Work out the finished part from the listing and answer in its coordinate system (mm). A direction names the side the tool comes from. Give positions to 0.01 mm unless a question says otherwise; leave off trailing zeros. Loops run counter-clockwise (first coordinate to the right, second up) from the corner with the lowest first, then second, coordinate; pieces in that order, holes last. Notation, with made-up numbers: (-7, -1.5) - (33, -1.5) arc R22 cw to (33, 26.5) - close; hole circle Ø8 at (88.25, 13.5). An arc over 180 degrees is marked (long way). Use CSV: the item, a comma, the result in double quotes.
from build123d import *

# Parameters (mm, degrees)
SKETCH_1_W       = 20
SKETCH_1_H       = 10
BASEPLATE_DEPTH  = 1
HEM_OPEN_DEPTH   = 20
HEM_OPEN_2_DEPTH = 20


# Read off the part's stored shape, not the designer's step: Hem_open
# Sheet-metal steps are written as plain solids
with BuildPart() as part:
    # Sketch 1 → BasePlate (new body)
    with BuildSketch(Plane.XY):
        with Locations((10, 5)):
            Rectangle(SKETCH_1_W, SKETCH_1_H)
    extrude(amount=-BASEPLATE_DEPTH)

    # Hem_open outline → Hem_open (cut)
    with BuildSketch(Plane.YZ):
        with BuildLine():
            Line((10, 0), (9.914213562, 0))
            ThreePointArc((9.914213562, 0), (9.366025404, -0.724744871), (8.5, -1))
            Line((8.5, -1), (10, -1))
            Line((10, -1), (10, 0))
        make_face()
    extrude(amount=HEM_OPEN_DEPTH, mode=Mode.SUBTRACT)

    # Hem_open 2 outline → Hem_open 2 (add)
    with BuildSketch(Plane.YZ):
        with BuildLine():
            Line((5, 2), (5, 1))
            Line((5, 1), (8.5, 1))
            ThreePointArc((8.5, 1), (9, 0.5), (8.5, 0))
            Line((8.5, 0), (9.914213562, 0))
            ThreePointArc((9.914213562, 0), (9.724744871, 1.366025404), (8.5, 2))
            Line((8.5, 2), (5, 2))
        make_face()
    extrude(amount=HEM_OPEN_2_DEPTH)


solid = part.part
Item 1: Find the intervals of material crossed by line 1 (Z direction, x = 3.25, y = 5.5); line 2 (Z direction, x = 2.25, y = 8.75); line 3 (Z direction, x = 6.25, y = 1), in increasing order.
Determined:
line 1,"z = -1 to 0, 1 to 2"
line 2,"z = -0.98 to 0.07, 0.93 to 1.98"
line 3,"z = -1 to 0"
Item 2: For faces 1 (the flat face through (10, 7, 1)), 2 (the flat face through (9.9, 5, 1.5)), 3 (the flat face through (10, 7, 2)), determine the directions among +Z, -Z, +X, -X, +Y, -Y from which every point of the face is accessible in a straight line to the end or side of a thin tool.
Determined:
face 1,"+X, -X, -Y"
face 2,"+Z, +X, -X, -Y"
face 3,"+Z, +X, -X, +Y, -Y"
Item 3: A cutting plane is placed at B-B on x = 2.25. Determine the outline of the cut face in (y, z), and give its area (3 significant figures).
Determined:
outline,"(0, -1) - (8.5, -1) arc R1.5 ccw to (8.5, 2) - (5, 2) - (5, 1) - (8.5, 1) arc R0.5 cw to (8.5, 0) - (0, 0) - close"
area,"15.1 mm²"
Item 4: A cutting plane is placed at C-C on y = 1.5. Determine the outline of the cut face in (x, z).
Determined:
outline,"(0, -1) - (20, -1) - (20, 0) - (0, 0) - close"
Item 5: The mould has two halves that part along Z. Classify faces 4 (the flat face through (10, 4, -1)), 5 (the flat face through (10, 4, 0)), 6 (the flat face through (9.9, 0, -0.5)): pulls with the +Z half, pulls with the -Z half, needs draft (parallel to the pull), parting line crosses it, or undercut.
Determined:
face 4,"pulls with the -Z half"
face 5,"undercut"
face 6,"needs draft"
Item 6: A cutting plane is placed at A-A on y = 5.75. Determine the outline of the cut face in (x, z).
Determined:
outline,"(0, -1) - (20, -1) - (20, 0) - (0, 0) - close; (0, 1) - (20, 1) - (20, 2) - (0, 2) - close"
Item 7: A cutting plane is placed at D-D on z = 0.5. Determine the outline of the cut face in (x, y).
Determined:
outline,"(0, 9) - (20, 9) - (20, 10) - (0, 10) - close"
Item 8: Given P1, Ø2.5, axis at x = 10, y = 4.5, coming from the +Z side, flat-ended and moving along its own axis, determine where the tip first touches the part or whether it passes through.
Determined:
P1,"stops at z = 2"
